Could you check a few things on this model? Use its own coordinates, in mm. A direction names the side the tool comes from. Give positions to 0.01 mm unless a question says otherwise; leave off trailing zeros. Write each loop counter-clockwise with the first axis right and the second up, starting at its lowest first coordinate (ties: lowest second). Pieces come first, ordered by that corner, then holes. Notation, with made-up numbers: (59, 17) - (69, 17) arc R19 cw to (69, 32) - close; hole circle Ø3 at (87, -29). An arc over 180 degrees is marked (long way). Use one line per item in the form item = value.
```python
from build123d import *

# Parameters (mm, degrees)
CUBE003_W                   = 50
CUBE003_H                   = 2
CUBE003_DEPTH               = 5
CYLINDER_R                  = 4.1
CYLINDER_DEPTH              = 13.8
CUBE004_W                   = 10
CUBE004_H                   = 10
CUBE004_DEPTH               = 20
CUBE004_PLACEMENT_ANGLE     = 45
CUBE005_W                   = 10
CUBE005_H                   = 10
CUBE005_DEPTH               = 20
CUBE005_PLACEMENT_ANGLE     = 45
CUBE006_W                   = 10
CUBE006_H                   = 10
CUBE006_DEPTH               = 20
CUBE006_PLACEMENT_ANGLE     = 45
CUBE007_W                   = 10
CUBE007_H                   = 10
CUBE007_DEPTH               = 20
CUBE007_PLACEMENT_ANGLE     = 45
CYLINDER001_R               = 3.1
CYLINDER001_DEPTH           = 10
CYLINDER002_R               = 3.1
CYLINDER002_DEPTH           = 10
CUBE008_W                   = 30
CUBE008_H                   = 2.1
CUBE008_DEPTH               = 3.5
CUBE002_W                   = 50
CUBE002_H                   = 2
CUBE002_DEPTH               = 10
CUBE001_W                   = 16
CUBE001_H                   = 17.5
CUBE001_DEPTH               = 18
CUBE_W                      = 42
CUBE_H                      = 7
CUBE_DEPTH                  = 18
DIFFERENCE_PLACEMENT_ANGLE  = 180
BASEFEATURE_PLACEMENT_ANGLE = 180
SKETCH_W                    = 13
SKETCH_H                    = 8
POCKET_DEPTH                = 0.5
SKETCH001_W                 = 16
SKETCH001_H                 = 8
PAD_DEPTH                   = 1
CHAMFER_SIZE                = 1.49


with BuildPart() as cube003:
    # cube003 → cube003 (new body)
    with BuildSketch(Plane(origin=(42.1, 0.5, 0), x_dir=(-1, 0, 0), z_dir=(0, 0, 1))):
        with Locations((25, 1)):
            Rectangle(CUBE003_W, CUBE003_H)
    extrude(amount=CUBE003_DEPTH)


with BuildPart() as cylinder:
    # cylinder → cylinder (new body)
    with BuildSketch(Plane(origin=(21, 15.9, -0.1), x_dir=(1, 0, 0), z_dir=(0, 0, 1))):
        Circle(CYLINDER_R)
    extrude(amount=CYLINDER_DEPTH)


with BuildPart() as cube004:
    # cube004 → cube004 (new body)
    with BuildSketch(Plane.XY):
        with Locations((5, 5)):
            Rectangle(CUBE004_W, CUBE004_H)
    extrude(amount=CUBE004_DEPTH)


with BuildPart() as cube004_1:
    # cube004 placement: moved
    add(cube004.part.moved(Location((13, 15.5, -0.1))).rotate(Axis((13, 15.5, -0.1), (0, 0, 1)), CUBE004_PLACEMENT_ANGLE))


with BuildPart() as cube005:
    # cube005 → cube005 (new body)
    with BuildSketch(Plane.XY):
        with Locations((5, 5)):
            Rectangle(CUBE005_W, CUBE005_H)
    extrude(amount=CUBE005_DEPTH)


with BuildPart() as cube005_1:
    # cube005 placement: moved
    add(cube005.part.moved(Location((29, 15.5, -0.1))).rotate(Axis((29, 15.5, -0.1), (0, 0, 1)), CUBE005_PLACEMENT_ANGLE))


with BuildPart() as cube006:
    # cube006 → cube006 (new body)
    with BuildSketch(Plane.XY):
        with Locations((5, 5)):
            Rectangle(CUBE006_W, CUBE006_H)
    extrude(amount=CUBE006_DEPTH)


with BuildPart() as cube006_1:
    # cube006 placement: moved
    add(cube006.part.moved(Location((0, 5.5, -0.1))).rotate(Axis((0, 5.5, -0.1), (0, 0, 1)), CUBE006_PLACEMENT_ANGLE))


with BuildPart() as cube007:
    # cube007 → cube007 (new body)
    with BuildSketch(Plane.XY):
        with Locations((5, 5)):
            Rectangle(CUBE007_W, CUBE007_H)
    extrude(amount=CUBE007_DEPTH)


with BuildPart() as cube007_1:
    # cube007 placement: moved
    add(cube007.part.moved(Location((42, 5.5, -0.1))).rotate(Axis((42, 5.5, -0.1), (0, 0, 1)), CUBE007_PLACEMENT_ANGLE))


with BuildPart() as cylinder001:
    # cylinder001 → cylinder001 (new body)
    with BuildSketch(Plane(origin=(6, -0.1, 9), x_dir=(1, 0, 0), z_dir=(0, 1, 0))):
        Circle(CYLINDER001_R)
    extrude(amount=CYLINDER001_DEPTH)


with BuildPart() as cylinder002:
    # cylinder002 → cylinder002 (new body)
    with BuildSketch(Plane(origin=(36, -0.1, 9), x_dir=(1, 0, 0), z_dir=(0, 1, 0))):
        Circle(CYLINDER002_R)
    extrude(amount=CYLINDER002_DEPTH)


with BuildPart() as cube008:
    # cube008 → cube008 (new body)
    with BuildSketch(Plane(origin=(5, 8.3, 7), x_dir=(1, 0, 0), z_dir=(0, 0, 1))):
        with Locations((15, 1.05)):
            Rectangle(CUBE008_W, CUBE008_H)
    extrude(amount=CUBE008_DEPTH)


with BuildPart() as group001:
    # cube002 → cube002 (new body)
    with BuildSketch(Plane(origin=(42.1, 0.5, 13), x_dir=(-1, 0, 0), z_dir=(0, 0, 1))):
        with Locations((25, 1)):
            Rectangle(CUBE002_W, CUBE002_H)
    extrude(amount=CUBE002_DEPTH)

    # Group001: union cube003, cylinder, cube004, cube005, cube006, cube007, cylinder001, cylinder002, cube008
    add(cube003.part)
    add(cylinder.part)
    add(cube004_1.part)
    add(cube005_1.part)
    add(cube006_1.part)
    add(cube007_1.part)
    add(cylinder001.part)
    add(cylinder002.part)
    add(cube008.part)


with BuildPart() as cube001:
    # cube001 → cube001 (new body)
    with BuildSketch(Plane(origin=(13, 0, 0), x_dir=(1, 0, 0), z_dir=(0, 0, 1))):
        with Locations((8, 8.75)):
            Rectangle(CUBE001_W, CUBE001_H)
    extrude(amount=CUBE001_DEPTH)


with BuildPart() as body:
    # cube → cube (new body)
    with BuildSketch(Plane.XY):
        with Locations((21, 3.5)):
            Rectangle(CUBE_W, CUBE_H)
    extrude(amount=CUBE_DEPTH)

    # Group: union cube001
    add(cube001.part)

    # difference: cut Group001
    add(group001.part, mode=Mode.SUBTRACT)


with BuildPart() as body_1:
    # difference placement: moved
    add(body.part.moved(Location((0, 0, 18))).rotate(Axis((0, 0, 18), (0, 1, 0)), DIFFERENCE_PLACEMENT_ANGLE))


with BuildPart() as body_2:
    # BaseFeature placement: moved
    add(body_1.part.moved(Location((0, 0, 18))).rotate(Axis((0, 0, 18), (0, -1, 0)), BASEFEATURE_PLACEMENT_ANGLE))

    # Sketch (on Face13 of BaseFeature) → Pocket (cut)
    with BuildSketch(Plane.XZ):
        with Locations((6.5, 9)):
            Rectangle(SKETCH_W, SKETCH_H)
        with Locations((35.5, 9)):
            Rectangle(SKETCH_W, SKETCH_H)
    extrude(amount=-POCKET_DEPTH, mode=Mode.SUBTRACT)

    # Sketch001 (on Face19 of Pocket) → Pad (join)
    with BuildSketch(Plane.XZ):
        with Locations((21, 9)):
            Rectangle(SKETCH001_W, SKETCH001_H)
    extrude(amount=PAD_DEPTH)

    # Chamfer
    chamfer_edges = [body_2.edges().sort_by_distance(p)[0] for p in [
        (21, -1, 13),
    ]]
    chamfer(chamfer_edges, length=CHAMFER_SIZE)


solid = body_2.part
```
1. Imagine slicing it at C-C, the plane z = 10. State how many separate pieces and enclosed holes the cut face has, and give its area (3 significant figures).
Response values:
separate_pieces = 4
enclosed_holes = 0
area = 310 mm²
2. Imagine slicing it at A-A, the plane x = 36. List the corners of the cut face in (y, z) for me.
Response values:
outline = (0.5, 0) - (7, 0) - (7, 5.9) - (0.5, 5.9) - close; (0.5, 12.1) - (7, 12.1) - (7, 18) - (0.5, 18) - close
3. If we mould it in two halves opening along Y, with no side actions, what happens to faces 1 (the face through (20.89, -0.27, 12.24)), 2 (the face through (21, 9, 10.5)), 3 (the face through (3.72, 3.7, 6.9)), 4 (the face through (17, 17.5, 11))? For each: pulls with the +Y half, pulls with the -Y half, needs draft (parallel to the pull), parting line crosses it, or undercut.
Response values:
face_1 = pulls with the -Y half
face_2 = undercut
face_3 = needs draft
face_4 = pulls with the +Y half
4. If I drill on line 1 (Z direction, x = 17.5, y = 9.25); line 2 (Z direction, x = 6, y = 2.5); line 3 (Y direction, x = 24, z = 17), over which ranges is the centre line in solid material (lowest first)? Write a range as from..to.
Response values:
line_1 = 0..7, 10.5..18
line_2 = 0..5.9, 12.1..18
line_3 = 0.5..17.5
5. Which directions (+Z, -Z, +X, -X, +Y, -Y) give clear straight access to the entire face, cutting with the end or side of a thin tool? Please do faces 5 (the face through (20.9, 11.8, 6.8)), 6 (the face through (21, 0, 5)), 7 (the face through (21, 10.4, 9)).
Response values:
face_5 = -Z
face_6 = -Z, +X, -X, -Y
face_7 = +X, -X
6. For pin 1 (4 mm diameter, centred on y = 13.5, z = 3.5, fed in from +X); pin 2 (1.5 mm diameter, centred on x = 34, z = 11.5, fed in from -Y); pin 3 (3 mm diameter, centred on x = 22, z = 8, fed in from +Y); pin 4 (3.5 mm diameter, centred on x = 6, z = 9, fed in from -Y), each with a flat end and sliding along its axis, tell me the tip position at first contact or that it passes through.
Response values:
pin_1 = 29
pin_2 = 0.5
pin_3 = 12.65
pin_4 = through
7. Imagine slicing it at B-B, the plane y = 3.5. List the corners of the cut face in (x, z) for me, and give its area (3 significant figures).
Response values:
outline = (0, 0) - (42, 0) - (42, 18) - (0, 18) - close; hole circle Ø6.2 at (6, 9); hole circle Ø6.2 at (36, 9)
area = 696 mm²
8. Imagine slicing it at D-D, the plane y = 15.9. List the corners of the cut face in (x, z) for me.
Response values:
outline = (13.4, 0) - (16.9, 0) - (16.9, 13.7) - (25.1, 13.7) - (25.1, 0) - (28.6, 0) - (28.6, 18) - (13.4, 18) - close
